Geometry check sheet. Reference: the model listing, model coordinates, mm. A direction names the side the tool comes from. Round coordinates to 2 decimals unless told otherwise and drop trailing zeros.
```python
from build123d import *

# Parameters (mm, degrees)
F1_DEPTH = 6.35


with BuildPart() as f1:
    # F0 (on Right) → F1 (new body)
    with BuildSketch(Plane.YZ):
        Polygon((64.29375, 28.575), (-51.59375, 28.575), (-51.59375, 22.225), (-64.29375, 22.225), (-64.29375, 15.875), (-51.59375, 15.875), (-51.59375, 9.525), (-64.29375, 9.525), (-64.29375, 3.175), (-51.59375, 3.175), (-51.59375, -3.175), (-64.29375, -3.175), (-64.29375, -9.525), (-51.59375, -9.525), (-51.59375, -15.875), (-64.29375, -15.875), (-64.29375, -22.225), (-51.59375, -22.225), (-51.59375, -28.575), (64.29375, -28.575), align=None)
        Polygon((180.18125, 28.575), (64.29375, 28.575), (64.29375, -28.575), (180.18125, -28.575), (180.18125, -22.225), (192.88125, -22.225), (192.88125, -15.875), (180.18125, -15.875), (180.18125, -9.525), (192.88125, -9.525), (192.88125, -3.175), (180.18125, -3.175), (180.18125, 3.175), (192.88125, 3.175), (192.88125, 9.525), (180.18125, 9.525), (180.18125, 15.875), (192.88125, 15.875), (192.88125, 22.225), (180.18125, 22.225), align=None)
    extrude(amount=F1_DEPTH)


solid = f1.part
```
(1) Depth check by flat-ended pin: P1, Ø1.9, axis at x = 4.5, y = 188.5, coming from the +Z side (3 decimals); P2, Ø2, axis at x = 1.5, z = -11.5, coming from the +Y side; P3, Ø3, axis at x = 1.5, y = -59.5, coming from the -Z side (3 decimals). Enter the tip coordinate at first touch or a pass-through.
Returned:
P1: stops at z = 22.225
P2: stops at y = 180.18
P3: stops at z = -22.225
(2) Material ranges on line 1 (Y direction, x = 2.25, z = 23), recorded low to high.
Returned:
line 1: y = -51.59 to 180.18
(3) Set-up check for faces 1 (the flat face through (3, -58, 22.225)), 2 (the flat face through (3, -58, 9.525)), 3 (the flat face through (3, -51.594, -25)): record each of +Z, -Z, +X, -X, +Y, -Y from which the full face is reachable in a straight line by a thin tool's end or side.
Returned:
face 1: +Z, +X, -X, -Y
face 2: +X, -X, -Y
face 3: -Z, +X, -X, -Y
